```python
from build123d import *

# Parameters (mm, degrees)
SKETCH1_W           = 54.5
SKETCH1_H           = 34.5
BOSS_EXTRUDE1_DEPTH = 1.5
SKETCH6_W           = 5
SKETCH6_H           = 14.5
CUT_EXTRUDE1_DEPTH  = 2
SKETCH9_W           = 5
SKETCH9_H           = 14.5
CUT_EXTRUDE2_DEPTH  = 2
SKETCH27_W          = 1.5
SKETCH27_H          = 10
CUT_EXTRUDE3_DEPTH  = 2
SKETCH37_W          = 1.5
SKETCH37_H          = 10
CUT_EXTRUDE10_DEPTH = 2
SKETCH39_W          = 1.5
SKETCH39_H          = 10
CUT_EXTRUDE11_DEPTH = 2
SKETCH41_W          = 1.5
SKETCH41_H          = 10
CUT_EXTRUDE12_DEPTH = 2


with BuildPart() as part:
    # Sketch1 → Boss-Extrude1 (new body)
    with BuildSketch(Plane(origin=(0, 0, 0), x_dir=(1, 0, 0), z_dir=(0, 1, 0))):
        Rectangle(SKETCH1_W, SKETCH1_H)
    extrude(amount=BOSS_EXTRUDE1_DEPTH)

    # Sketch6 → Cut-Extrude1 (cut)
    with BuildSketch(Plane(origin=(0, 1.5, 0), x_dir=(1, 0, 0), z_dir=(0, 1, 0))):
        with Locations((-12.75, 6)):
            Rectangle(SKETCH6_W, SKETCH6_H)
    extrude(amount=-CUT_EXTRUDE1_DEPTH, mode=Mode.SUBTRACT)

    # Sketch9 → Cut-Extrude2 (cut)
    with BuildSketch(Plane(origin=(0, 1.5, 0), x_dir=(1, 0, 0), z_dir=(0, 1, 0))):
        with Locations((12.75, 6)):
            Rectangle(SKETCH9_W, SKETCH9_H)
    extrude(amount=-CUT_EXTRUDE2_DEPTH, mode=Mode.SUBTRACT)

    # Sketch27 → Cut-Extrude3 (cut)
    with BuildSketch(Plane(origin=(0, 1.5, 0), x_dir=(1, 0, 0), z_dir=(0, 1, 0))):
        with Locations((-21, -12.25)):
            Rectangle(SKETCH27_W, SKETCH27_H)
    extrude(amount=-CUT_EXTRUDE3_DEPTH, mode=Mode.SUBTRACT)

    # Sketch37 → Cut-Extrude10 (cut)
    with BuildSketch(Plane(origin=(0, 1.5, 0), x_dir=(1, 0, 0), z_dir=(0, 1, 0))):
        with Locations((3.5, -12.25)):
            Rectangle(SKETCH37_W, SKETCH37_H)
    extrude(amount=-CUT_EXTRUDE10_DEPTH, mode=Mode.SUBTRACT)

    # Sketch39 → Cut-Extrude11 (cut)
    with BuildSketch(Plane(origin=(0, 1.5, 0), x_dir=(1, 0, 0), z_dir=(0, 1, 0))):
        with Locations((-8.75, -12.25)):
            Rectangle(SKETCH39_W, SKETCH39_H)
    extrude(amount=-CUT_EXTRUDE11_DEPTH, mode=Mode.SUBTRACT)

    # Sketch41 → Cut-Extrude12 (cut)
    with BuildSketch(Plane(origin=(0, 1.5, 0), x_dir=(1, 0, 0), z_dir=(0, 1, 0))):
        with Locations((15.75, -12.25)):
            Rectangle(SKETCH41_W, SKETCH41_H)
    extrude(amount=-CUT_EXTRUDE12_DEPTH, mode=Mode.SUBTRACT)


solid = part.part
```
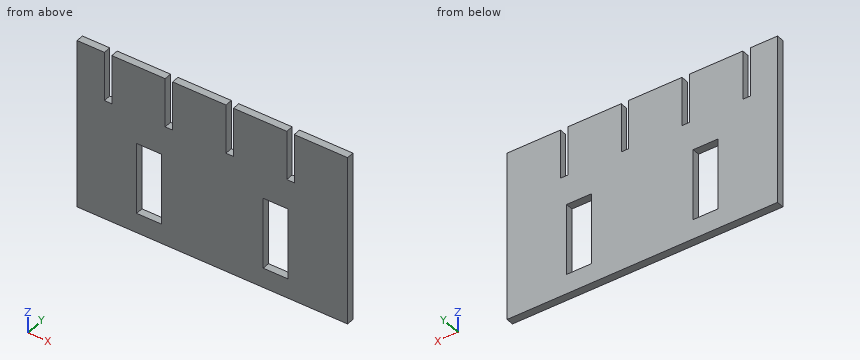
Geometry: final body of the model. Coordinates: model frame, mm. Coordinates: 2 decimals unless noted, no trailing zeros. Order: outer loops, then holes, each group sorted by start corner. A loop starts at its lowest first (then second) coordinate and runs counter-clockwise, first axis right, second up. Notation, with made-up numbers: M 12.25,49.5 L 18.25,49.5 A29 ccw 18.25,77.5 Z; hole C -5,61 d5. An arc over 180 degrees is marked long. Answer in a Markdown table with one row per item. Add a question column.
Q1. Section query A-A on z = 11.5. Return the cut outline in (x, y), and give its area (4 significant figures).
Q2. Section query C-C on y = 0.55. Return the cut outline in (x, z), and give its area (3 significant figures).
Q3. Section query B-B on z = -5.5. Return the cut outline in (x, y).
Q4. Line query: L1, parallel to X at y = 0.9, z = -2.5; L2, parallel to X at y = 0.7, z = 14; L3, parallel to Z at x = -11.5, y = 1.4. Output: solid intervals per line, ascending.
Completed:
| question | item | result |
|---|---|---|
| 1 | outline | M -27.25,0 L -21.75,0 L -21.75,1.5 L -27.25,1.5 Z; M -20.25,0 L -9.5,0 L -9.5,1.5 L -20.25,1.5 Z; M -8,0 L 2.75,0 L 2.75,1.5 L -8,1.5 Z; M 4.25,0 L 15,0 L 15,1.5 L 4.25,1.5 Z; M 16.5,0 L 27.25,0 L 27.25,1.5 L 16.5,1.5 Z |
| 1 | area | 72.75 mm2 |
| 2 | outline | M -27.25,-17.25 L 27.25,-17.25 L 27.25,17.25 L 16.5,17.25 L 16.5,7.25 L 15,7.25 L 15,17.25 L 4.25,17.25 L 4.25,7.25 L 2.75,7.25 L 2.75,17.25 L -8,17.25 L -8,7.25 L -9.5,7.25 L -9.5,17.25 L -20.25,17.25 L -20.25,7.25 L -21.75,7.25 L -21.75,17.25 L -27.25,17.25 Z; hole M -15.25,-13.25 L -10.25,-13.25 L -10.25,1.25 L -15.25,1.25 Z; hole M 10.25,-13.25 L 15.25,-13.25 L 15.25,1.25 L 10.25,1.25 Z |
| 2 | area | 1,680 mm2 |
| 3 | outline | M -27.25,0 L -15.25,0 L -15.25,1.5 L -27.25,1.5 Z; M -10.25,0 L 10.25,0 L 10.25,1.5 L -10.25,1.5 Z; M 15.25,0 L 27.25,0 L 27.25,1.5 L 15.25,1.5 Z |
| 4 | L1 | x = -27.25 to -15.25, -10.25 to 10.25, 15.25 to 27.25 |
| 4 | L2 | x = -27.25 to -21.75, -20.25 to -9.5, -8 to 2.75, 4.25 to 15, 16.5 to 27.25 |
| 4 | L3 | z = -17.25 to -13.25, 1.25 to 17.25 |
